Autodesk Inventor part; units mm, degrees
ref_plane "YZ Plane" through (0, 0, 0) normal (1, 0, 0) x (0, 1, 0)
ref_plane "XZ Plane" through (0, 0, 0) normal (0, 1, 0) x (-1, 0, 0)
ref_plane "XY Plane" through (0, 0, 0) normal (0, 0, 1) x (1, 0, 0)
sketch "Sketch2" plane through (0, 0, 0) normal (1, 0, 0) x (0, 1, 0)
  circle A0 centre (0, 0) radius 31.85 construction
  circle A1 centre (0, 64.66) radius 12.75 construction
  line L0 (12.181, 68.4262) -> (30.4287, 9.4082)
  line L1 (-12.181, 68.4262) -> (-30.4287, 9.4082)
  arc A2 (12.181, 68.4262) -> (-12.181, 68.4262) centre (0, 64.66) ccw
  arc A3 (-30.4287, 9.4082) -> (30.4287, 9.4082) centre (0, 0) ccw
  line L2 (31.5179, 9.745) -> (13.2702, 68.763)
  arc A4 (13.2702, 68.763) -> (-13.2702, 68.763) centre (0, 64.66) ccw
  line L3 (-13.2702, 68.763) -> (-31.5179, 9.745)
  arc A5 (-31.5179, 9.745) -> (31.5179, 9.745) centre (0, 0) ccw
  dimension "d0" = 63.7
  dimension "d1" = 25.5
  dimension "d2" = 64.66
  dimension "d3" = 1.14
extrude "Extrusion1" add sketch "Sketch2" along normal mid plane 9
properties part number "TimingBlet" material "Rubber"
Build history of the part. All positions in model axes, mm. A direction names the side the tool comes from. Give positions to 0.01 mm unless a question says otherwise; leave off trailing zeros. Loops run counter-clockwise (first coordinate to the right, second up) from the corner with the lowest first, then second, coordinate; pieces in that order, holes last. Notation, with made-up numbers: (10.25, 14.25) -> (55.25, 14.25) arc R28 cw to (55.25, 36.25) -> close; hole circle Ø1 at (23.25, 36). An arc over 180 degrees is marked (long way). Answer in a Markdown table with one row per item.
Item 1: Mould opens along Y. For faces 3 (the cylindrical face through (-0.06, 0.86, -32.98)), 4 (the flat face through (-0.06, 22.52, 38.84)), 5 (the flat face through (-0.063, -21.177, 39.33)) say: pulls with the +Y half, pulls with the -Y half, needs draft (parallel to the pull), parting line crosses it, or undercut.
Findings below:
| item | result |
|---|---|
| face 3 | parting line crosses it |
| face 4 | pulls with the +Y half |
| face 5 | undercut |
Item 2: Flat gauge pins, fed straight in: P1, Ø1, axis at x = 1, z = 33, coming from the +Y side; P2, Ø10, axis at y = -7, z = 62, coming from the +X side; P3, Ø1.5, axis at x = -0.5, z = -1, coming from the -Y side. Where does each tip first touch, or does it go through?
Findings below:
| item | result |
|---|---|
| P1 | stops at y = 24.48 |
| P2 | passes through |
| P3 | stops at y = -32.99 |
Item 3: Slice it at C-C on x = -1. Write the cut outline in (y, z) (3 decimals), plus the area to 3 significant figures.
Findings below:
| item | result |
|---|---|
| outline | (-31.518, 9.745) arc R32.99 ccw (long way) to (31.518, 9.745) -> (13.27, 68.763) arc R13.89 ccw to (-13.27, 68.763) -> close; hole (-30.429, 9.408) arc R31.85 ccw (long way) to (30.429, 9.408) -> (12.181, 68.426) arc R12.75 ccw to (-12.181, 68.426) -> close |
| area | 318 mm² |
Item 4: Slice it at A-A on z = 0. Write the cut outline in (x, y).
Findings below:
| item | result |
|---|---|
| outline | (-4.5, -32.99) -> (4.5, -32.99) -> (4.5, -31.85) -> (-4.5, -31.85) -> close; (-4.5, 31.85) -> (4.5, 31.85) -> (4.5, 32.99) -> (-4.5, 32.99) -> close |
Item 5: Slice it at B-B on y = 18.5. Write the cut outline in (x, z).
Findings below:
| item | result |
|---|---|
| outline | (-4.5, -27.31) -> (4.5, -27.31) -> (4.5, -25.93) -> (-4.5, -25.93) -> close; (-4.5, 47.99) -> (4.5, 47.99) -> (4.5, 51.85) -> (-4.5, 51.85) -> close |
Item 6: Probe line 1 along Z through (x, y) = (0.25, 0); line 2 along Y through (x, z) = (-1.75, 0); line 3 along Z through (x, y) = (1, -11). List the from-to ranges inside material, lowest first. Write a range as [from, to].
Findings below:
| item | result |
|---|---|
| line 1 | z = [-32.99, -31.85], [77.41, 78.55] |
| line 2 | y = [-32.99, -31.85], [31.85, 32.99] |
| line 3 | z = [-31.1, -29.89], [71.11, 73.14] |
Item 7: Tool access for faces 1 (the cylindrical face through (-0.063, -0.227, 77.408)), 2 (the flat face through (-4.5, -27, 23)): list every direction of +Z, -Z, +X, -X, +Y, -Y with a clear straight run to the whole face (end or side of a thin tool).
Findings below:
| item | result |
|---|---|
| face 1 | +X, -X |
| face 2 | +Z, -Z, -X, +Y, -Y |
